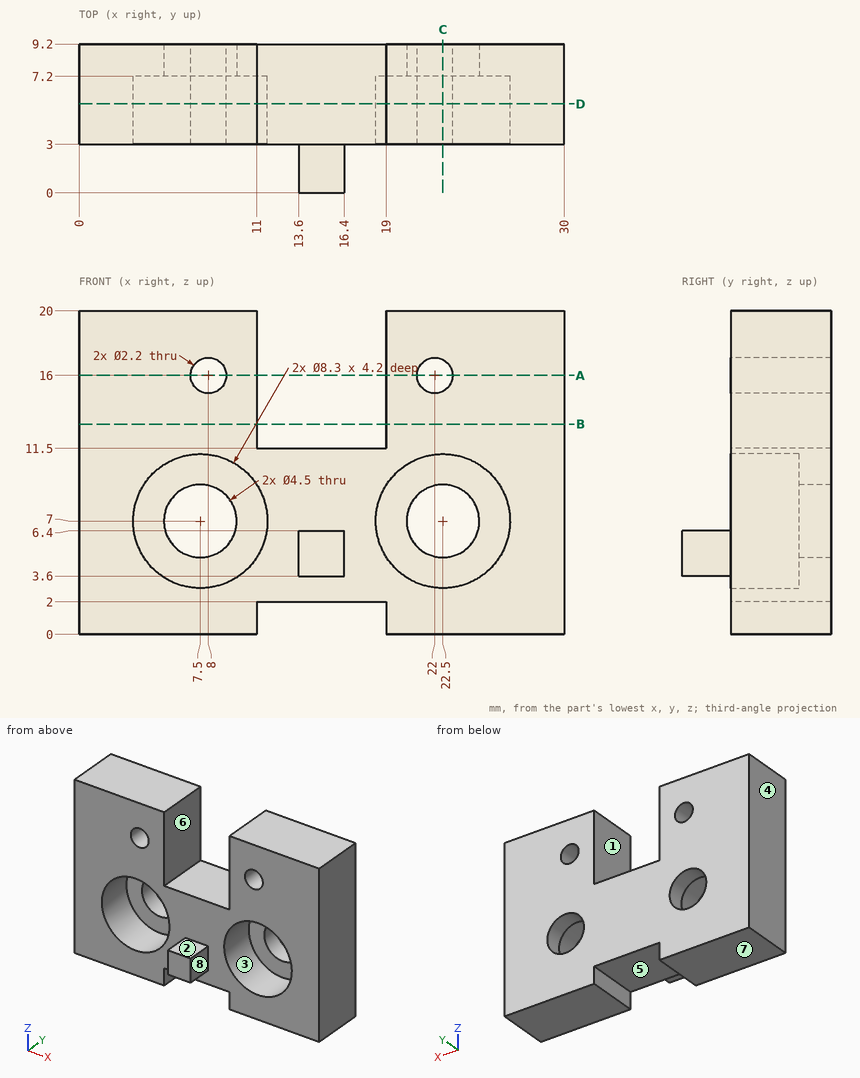
Check sheet for the drawn part. Datum: minimum x, y, z corner. Units: mm. A direction names the side the tool comes from. Coordinates: 2 decimals unless noted, no trailing zeros. Loops run counter-clockwise (first coordinate to the right, second up) from the corner with the lowest first, then second, coordinate; pieces in that order, holes last. Notation, with made-up numbers: (-32.5, 64.5) -> (-10.5, 64.5) arc R25 cw to (-10.5, 90.5) -> close; hole circle Ø5 at (77, -27). An arc over 180 degrees is marked (long way). Answer in a Markdown table with one row per item.
1. Material ranges on line 1 along X through (y, z) = (8.2, 7); line 2 along Z through (x, y) = (8.25, 8.5); line 3 along X through (y, z) = (8.5, 16.75), recorded low to high. Write a range as [from, to].
Check values:
| item | result |
|---|---|
| line 1 | x = [0, 5.25], [9.75, 20.25], [24.75, 30] |
| line 2 | z = [0, 4.88], [9.12, 14.93], [17.07, 20] |
| line 3 | x = [0, 7.2], [8.8, 11], [19, 21.2], [22.8, 30] |
2. Access from +Z, -Z, +X, -X, +Y, -Y to the whole of each face (thin tool, end or side, straight path). Record for the marked faces 1, 2, 3, 4 and 5.
Check values:
| item | result |
|---|---|
| face 1 | +Z, +Y, -Y |
| face 2 | +Z, +X, -X, -Y |
| face 3 | -Y |
| face 4 | +Z, -Z, -X, +Y, -Y |
| face 5 | -Z, +Y, -Y |
3. Sectioned sample at A-A, the plane z = 16. Record the boundary of the cut face in (x, y), then the cut area to 3 significant figures.
Check values:
| item | result |
|---|---|
| outline | (0, 3) -> (6.9, 3) -> (6.9, 9.2) -> (0, 9.2) -> close; (9.1, 3) -> (11, 3) -> (11, 9.2) -> (9.1, 9.2) -> close; (19, 3) -> (20.9, 3) -> (20.9, 9.2) -> (19, 9.2) -> close; (23.1, 3) -> (30, 3) -> (30, 9.2) -> (23.1, 9.2) -> close |
| area | 109 mm2 |
4. Sectioned sample at C-C, the plane x = 22.5. Record the boundary of the cut face in (y, z).
Check values:
| item | result |
|---|---|
| outline | (3, 0) -> (9.2, 0) -> (9.2, 4.75) -> (7.2, 4.75) -> (7.2, 2.85) -> (3, 2.85) -> close; (3, 11.15) -> (7.2, 11.15) -> (7.2, 9.25) -> (9.2, 9.25) -> (9.2, 15.02) -> (3, 15.02) -> close; (3, 16.98) -> (9.2, 16.98) -> (9.2, 20) -> (3, 20) -> close |
5. Release check for a two-part mould opening along X. For the marked faces 6, 7 and 8 record: released by +X, released by -X, zero draft, split by the parting line, or undercut.
Check values:
| item | result |
|---|---|
| face 6 | undercut |
| face 7 | zero draft |
| face 8 | released by +X |
6. Sectioned sample at B-B, the plane z = 13. Record the boundary of the cut face in (x, y), then the cut area to 3 significant figures.
Check values:
| item | result |
|---|---|
| outline | (0, 3) -> (11, 3) -> (11, 9.2) -> (0, 9.2) -> close; (19, 3) -> (30, 3) -> (30, 9.2) -> (19, 9.2) -> close |
| area | 136 mm2 |
7. Sectioned sample at D-D, the plane y = 5.5. Record the boundary of the cut face in (x, z), then the cut area to 3 significant figures.
Check values:
| item | result |
|---|---|
| outline | (0, 0) -> (11, 0) -> (11, 2) -> (19, 2) -> (19, 0) -> (30, 0) -> (30, 20) -> (19, 20) -> (19, 11.5) -> (11, 11.5) -> (11, 20) -> (0, 20) -> close; hole circle Ø8.3 at (7.5, 7); hole circle Ø2.2 at (8, 16); hole circle Ø8.3 at (22.5, 7); hole circle Ø2.2 at (22, 16) |
| area | 400 mm2 |
8. Go/stop test with flat-tipped pins: pin 1 (4 mm diameter, centred on x = 22.5, z = 8, fed in from -Y); pin 2 (5 mm diameter, centred on x = 11, z = 16, fed in from -Y); pin 3 (1.4 mm diameter, centred on x = 15, y = 1.5, fed in from +Z). Record where each tip stops, or that it passes through.
Check values:
| item | result |
|---|---|
| pin 1 | stops at y = 7.2 |
| pin 2 | stops at y = 3 |
| pin 3 | stops at z = 6.4 |
